Part model, mm, in its own coordinate system. Face numbers are marked on the shaded views. A direction names the side the tool comes from. Round coordinates to 2 decimals unless told otherwise and drop trailing zeros. Loops run counter-clockwise (first coordinate to the right, second up) from the corner with the lowest first, then second, coordinate; pieces in that order, holes last. Notation, with made-up numbers: M -12.5,57.25 L 0.5,57.25 A10 ccw 0.5,68.25 Z; hole C 63,65 d3. An arc over 180 degrees is marked long. Answer as CSV lines item,"result". Start each with the question number.
Item 1: Band-saw the part on A-A (y = 30.5). Give the cut face in (x, z), and give its area (3 significant figures).
Item 2: Drop flat-ended pins along their axis: pin 1 Ø1 at (y, z) = (51.5, -14) entering from -X; pin 2 Ø6 at (y, z) = (31.5, -21.5) entering from -X; pin 3 Ø2 at (x, z) = (-43.5, -18.5) entering from -Y. Give the stop position or say it passes through.
Item 3: Wall check: line 1 (Y direction, x = -44, z = -14.25); line 2 (Y direction, x = -42.5, z = -18); line 3 (Y direction, x = -45, z = -16). Give the ranges that are in metal, low to high.
Item 4: Which spindle directions (+Z, -Z, +X, -X, +Y, -Y) get a long thin tool onto all of the face, cutting with end or side? Do the marked faces 1 and 2. Say none if no direction does.
```python
from build123d import *

# Parameters (mm, degrees)
BOSS_EXTRUDE1_DEPTH = 10.6172
SKETCH2_R           = 5.588
BOSS_EXTRUDE2_DEPTH = 1.4986
BOSS_EXTRUDE3_DEPTH = 13.2842
SKETCH4_R           = 4.7498
BOSS_EXTRUDE4_DEPTH = 7.112
BOSS_EXTRUDE7_DEPTH = 134.62
SKETCH5_R           = 3.1623
BOSS_EXTRUDE5_DEPTH = 12.7
CHAMFER1_SIZE       = 0.508
CHAMFER2_SIZE       = 0.508
CUT_EXTRUDE2_START  = -59.4614
CUT_EXTRUDE2_DEPTH  = 59.4614
SKETCH12_R          = 5.9436
BOSS_EXTRUDE8_DEPTH = 0.9906
SKETCH13_R          = 6.35
BOSS_EXTRUDE9_DEPTH = 1.5875
CHAMFER3_SIZE       = 0.79375


with BuildPart() as part:
    # Sketch1 → Boss-Extrude1 (new body)
    with BuildSketch(Plane(origin=(0, 0, 0), x_dir=(1, 0, 0), z_dir=(0, 1, 0))):
        Polygon((-34.640959507, 23.019011646), (-41.973307925, 23.019011646), (-45.639482135, 16.669011646), (-41.973307925, 10.319011646), (-34.640959507, 10.319011646), (-30.974785297, 16.669011646), align=None)
    extrude(amount=-BOSS_EXTRUDE1_DEPTH)

    # Sketch2 → Boss-Extrude2 (add)
    with BuildSketch(Plane.XZ.offset(10.6172)):
        with Locations(Location((-38.307133716, -16.669011646, 0), (0, 0, 90))):
            Circle(SKETCH2_R)
    extrude(amount=BOSS_EXTRUDE2_DEPTH)

    # Sketch3 → Boss-Extrude3 (add)
    with BuildSketch(Plane(origin=(0, -12.1158, 0), x_dir=(-1, 0, 0), z_dir=(0, 1, 0))):
        Polygon((41.973307925, -23.019011646), (45.639482135, -16.669011646), (41.973307925, -10.319011646), (34.640959507, -10.319011646), (30.974785297, -16.669011646), (34.640959507, -23.019011646), align=None)
    extrude(amount=-BOSS_EXTRUDE3_DEPTH)

    # Sketch4 → Boss-Extrude4 (add)
    with BuildSketch(Plane.XZ.offset(25.4)):
        with Locations(Location((-38.307133716, -16.669011646, 0), (0, 0, 90))):
            Circle(SKETCH4_R)
    extrude(amount=BOSS_EXTRUDE4_DEPTH)

    # Sketch10 → Boss-Extrude7 (add)
    with BuildSketch(Plane(origin=(0, 0, 0), x_dir=(1, 0, 0), z_dir=(0, 1, 0))):
        Polygon((-30.974785297, 16.669011646), (-34.640959507, 23.019011646), (-41.973307925, 23.019011646), (-45.639482135, 16.669011646), (-41.973307925, 10.319011646), (-34.640959507, 10.319011646), align=None)
    extrude(amount=BOSS_EXTRUDE7_DEPTH)

    # Sketch5 → Boss-Extrude5 (add)
    with BuildSketch(Plane.XZ.offset(32.512)):
        with Locations(Location((-38.307133716, -16.669011646, 0), (0, 0, 270))):
            Circle(SKETCH5_R)
    extrude(amount=BOSS_EXTRUDE5_DEPTH)

    # Chamfer1
    chamfer1_edges = [part.edges().sort_by_distance(p)[0] for p in [
        (-38.307133716, -45.212, -13.506711646),
    ]]
    chamfer(chamfer1_edges, length=CHAMFER1_SIZE)

    # Chamfer2
    chamfer2_edges = [part.edges().sort_by_distance(p)[0] for p in [
        (-38.307133716, -32.512, -21.418811646),
    ]]
    chamfer(chamfer2_edges, length=CHAMFER2_SIZE)

    # Sketch11 → Cut-Extrude2 (cut)
    with BuildSketch(Plane(origin=(0, 134.62, 0), x_dir=(1, 0, 0), z_dir=(0, 1, 0)).offset(CUT_EXTRUDE2_START)):
        Polygon((-34.640959507, 10.319011646), (-30.974785297, 16.669011646), (-34.640959507, 23.019011646), (-41.973307925, 23.019011646), (-45.639482135, 16.669011646), (-41.973307925, 10.319011646), align=None)
    extrude(amount=CUT_EXTRUDE2_DEPTH, mode=Mode.SUBTRACT)

    # Sketch12 → Boss-Extrude8 (add)
    with BuildSketch(Plane(origin=(0, 75.1586, 0), x_dir=(1, 0, 0), z_dir=(0, 1, 0))):
        with Locations((-38.307133716, 16.669011646)):
            Circle(SKETCH12_R)
    extrude(amount=BOSS_EXTRUDE8_DEPTH)

    # Sketch13 → Boss-Extrude9 (add)
    with BuildSketch(Plane(origin=(0, 76.1492, 0), x_dir=(1, 0, 0), z_dir=(0, 1, 0))):
        with Locations(Location((-38.307133716, 16.669011646, 0), (0, 0, 180))):
            Circle(SKETCH13_R)
    extrude(amount=BOSS_EXTRUDE9_DEPTH)

    # Chamfer3
    chamfer3_edges = [part.edges().sort_by_distance(p)[0] for p in [
        (-31.957133716, 77.7367, -16.669011646),
    ]]
    chamfer(chamfer3_edges, length=CHAMFER3_SIZE)


solid = part.part
```
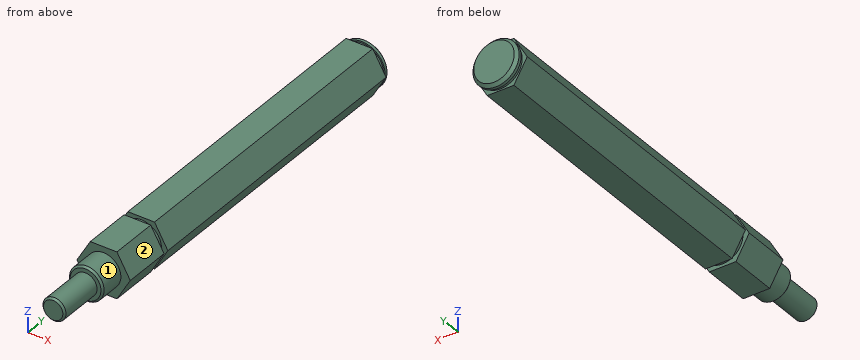
Answer block:
1,outline,"M -45.64,-16.67 L -41.97,-23.02 L -34.64,-23.02 L -30.97,-16.67 L -34.64,-10.32 L -41.97,-10.32 Z"
1,area,"140 mm^2"
2,pin 1,"stops at x = -44.39"
2,pin 2,"stops at x = -44.58"
2,pin 3,"stops at y = -32.25"
3,line 1,"y = -25.4 to -12.12, -10.62 to 75.16, 76.15 to 77.11"
3,line 2,"y = -32.35 to 77.74"
3,line 3,"y = -25.4 to -12.12, -10.62 to 75.16"
4,face 1,"-Y"
4,face 2,"+Z, +X, +Y, -Y"
